The drawing under review shows one solid part. Ordinate dimensions are in mm from its lowest x, y, z. A direction names the side the tool comes from. Give positions to 0.01 mm unless a question says otherwise; leave off trailing zeros. Write each loop counter-clockwise with the first axis right and the second up, starting at its lowest first coordinate (ties: lowest second). Pieces come first, ordered by that corner, then holes. Notation, with made-up numbers: (62.5, 63.5) -> (68.5, 63.5) arc R5 cw to (68.5, 72.5) -> close; hole circle Ø8 at (9, -16.75). An arc over 180 degrees is marked (long way). Answer as a JSON object with one key per item and string values.
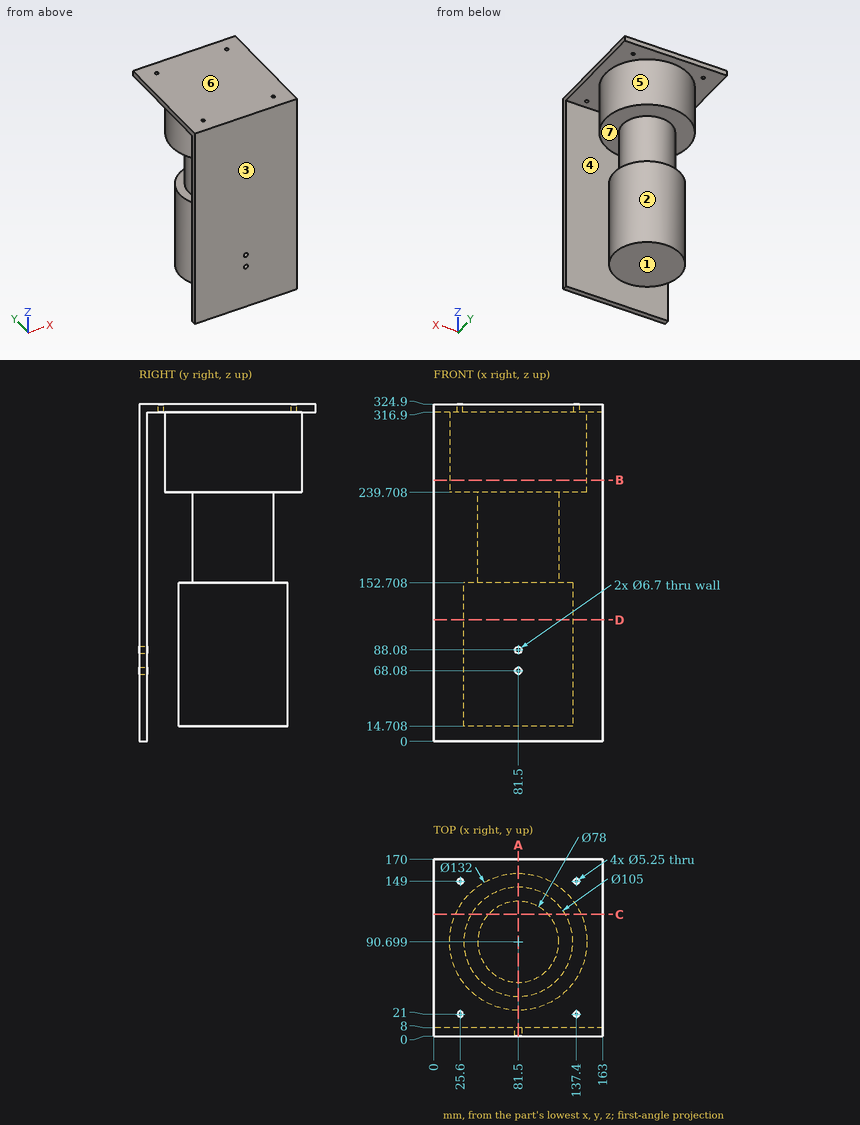
(1) Clearance check with flat-ended pins moving along their axes: pin 1 (4 mm diameter, centred on x = 25.6, y = 149, fed in from +Z); pin 2 (8.5 mm diameter, centred on x = 25.6, y = 21, fed in from -Z); pin 3 (12 mm diameter, centred on x = 58.5, z = 236, fed in from +Y); pin 4 (6 mm diameter, centred on x = 137.4, y = 21, fed in from +Z). State where each tip first meets the part, or that it passes through.
Here are the results:
{"pin 1": "passes through", "pin 2": "stops at z = 316.9", "pin 3": "stops at y = 154.12", "pin 4": "stops at z = 324.9"}
(2) For the marked faces 4, 5, 6 and 7, list the 3-axis set-ups (+Z, -Z, +X, -X, +Y, -Y) from which the entire face can be reached by the end or side of a thin tool; tool diameter is ignored.
Here are the results:
{"face 4": "-Z, +X, -X", "face 5": "-Z", "face 6": "+Z, +X, -X, +Y, -Y", "face 7": "none"}
(3) The part is to be moulded in two halves that separate along Y. For the marked faces 1, 2 and 3, say which applies: +Y half, -Y half, draft (parallel to the pull), parting line (faces both ways), or undercut.
Here are the results:
{"face 1": "draft", "face 2": "undercut", "face 3": "-Y half"}
(4) We need section D-D, the plane z = 117. State the section outline as (x, y) points.
Here are the results:
{"outline": "(0, 0) -> (163, 0) -> (163, 8) -> (0, 8) -> close; circle Ø105 at (81.5, 90.7)"}
(5) We need section A-A, the plane x = 81.5. State the section outline as (y, z) points.
Here are the results:
{"outline": "(0, 0) -> (8, 0) -> (8, 64.73) -> (0, 64.73) -> close; (0, 71.43) -> (8, 71.43) -> (8, 84.73) -> (0, 84.73) -> close; (0, 91.43) -> (8, 91.43) -> (8, 316.9) -> (24.7, 316.9) -> (24.7, 239.71) -> (51.7, 239.71) -> (51.7, 152.71) -> (38.2, 152.71) -> (38.2, 14.71) -> (143.2, 14.71) -> (143.2, 152.71) -> (129.7, 152.71) -> (129.7, 239.71) -> (156.7, 239.71) -> (156.7, 316.9) -> (170, 316.9) -> (170, 324.9) -> (0, 324.9) -> close"}
(6) For line 1 along X through (y, z) = (149, 321) (3 decimals); line 2 along Y through (x, z) = (25.6, 322) (3 decimals); line 3 along Z through (x, y) = (111.5, 62), list the stretches that pass through material, from the lowest coordinate up.
Here are the results:
{"line 1": "x = 0 to 22.975, 28.225 to 134.775, 140.025 to 163", "line 2": "y = 0 to 18.375, 23.625 to 146.375, 151.625 to 170", "line 3": "z = 14.71 to 152.71, 239.71 to 324.9"}
(7) We need section C-C, the plane y = 117. State the section outline as (x, z) points.
Here are the results:
{"outline": "(0, 316.9) -> (20.97, 316.9) -> (20.97, 239.71) -> (52.7, 239.71) -> (52.7, 152.71) -> (36.06, 152.71) -> (36.06, 14.71) -> (126.94, 14.71) -> (126.94, 152.71) -> (110.3, 152.71) -> (110.3, 239.71) -> (142.03, 239.71) -> (142.03, 316.9) -> (163, 316.9) -> (163, 324.9) -> (0, 324.9) -> close"}
(8) We need section B-B, the plane z = 251.5. State the section outline as (x, y) points, then the cut area to 3 significant figures.
Here are the results:
{"outline": "(0, 0) -> (163, 0) -> (163, 8) -> (0, 8) -> close; circle Ø132 at (81.5, 90.7)", "area": "15,000 mm²"}
